from build123d import *

# Parameters (mm, degrees)
SKETCH1_R               = 2
SKETCH1_R_2             = 5.5
SKETCH1_R_3             = 4
BOSS_EXTRUDE1_DEPTH     = 9
BOSS_EXTRUDE2_START     = -27
BOSS_EXTRUDE2_OUTLINE_R = 2
BOSS_EXTRUDE2_DEPTH     = 18
FILLET1_R               = 4
FILLET2_R               = 3
SKETCH3_R               = 11.25
CUT_EXTRUDE1_DEPTH      = 3.5
BOSS_EXTRUDE3_START     = -9
BOSS_EXTRUDE3_DEPTH     = 9
CUT_EXTRUDE2_DEPTH      = 93.793746104
CUT_EXTRUDE2_DEPTH_BACK = 93.793746104
SKETCH7_W               = 7.5
SKETCH7_H               = 5
CUT_EXTRUDE3_DEPTH      = 8.25
SKETCH8_R               = 2
CUT_EXTRUDE5_DEPTH      = 8.25
FILLET4_R               = 6


# Read off the part's stored shape, not the designer's step: Boss-Extrude2
with BuildPart() as part:
    # Sketch1 → Boss-Extrude1 (new body)
    with BuildSketch(Plane.XY):
        with BuildLine():
            Line((0, -15), (55.445040355, -15))
            ThreePointArc((55.445040355, -15), (77.945040355, 7.5), (55.445040355, 30))
            Line((55.445040355, 30), (12.958080577, 30))
            ThreePointArc((12.958080577, 30), (2.222427952, 26.874411477), (-5.157701411, 18.474576271))
            Line((-5.157701411, 18.474576271), (-11.322363742, 5.296610169))
            ThreePointArc((-11.322363742, 5.296610169), (-10.546507173, -6.709782891), (0, -12.5))
            Line((0, -12.5), (0, -15))
        make_face()
        with Locations((50.121730514, 23.802909935)):
            Circle(SKETCH1_R, mode=Mode.SUBTRACT)
        with Locations((60.768350196, -8.802909935)):
            Circle(SKETCH1_R, mode=Mode.SUBTRACT)
        with Locations((55.445040355, 7.5)):
            Circle(SKETCH1_R_2, mode=Mode.SUBTRACT)
        with Locations((71.74795029, 12.823309841)):
            Circle(SKETCH1_R, mode=Mode.SUBTRACT)
        Circle(SKETCH1_R_3, mode=Mode.SUBTRACT)
    extrude(amount=BOSS_EXTRUDE1_DEPTH)

    # Boss-Extrude2 outline → Boss-Extrude2 (add)
    with BuildSketch(Plane.XY.offset(9).offset(BOSS_EXTRUDE2_START)):
        with BuildLine():
            ThreePointArc((55.445040355, -15), (76.903671747, 14.265880489), (42.539570537, 25.930920997))
            Line((42.539570537, 25.930920997), (47.701758465, 18.558552598))
            ThreePointArc((47.701758465, 18.558552598), (68.32021919, 11.559528293), (55.445040355, -6))
            Line((55.445040355, -6), (55.445040355, -15))
        make_face()
        with Locations((60.768350196, -8.802909935)):
            Circle(BOSS_EXTRUDE2_OUTLINE_R, mode=Mode.SUBTRACT)
        with Locations((50.121730514, 23.802909935)):
            Circle(BOSS_EXTRUDE2_OUTLINE_R, mode=Mode.SUBTRACT)
        with Locations((71.74795029, 12.823309841)):
            Circle(BOSS_EXTRUDE2_OUTLINE_R, mode=Mode.SUBTRACT)
    extrude(amount=BOSS_EXTRUDE2_DEPTH)

    # Fillet1
    fillet1_edges = [part.edges().sort_by_distance(p)[0] for p in [
        (55.445040355, -6, -9),
        (55.445040355, -15, -9),
    ]]
    fillet(fillet1_edges, radius=FILLET1_R)

    # Fillet2
    fillet2_edges = [part.edges().sort_by_distance(p)[0] for p in [
        (47.701758465, 18.558552598, -9),
        (42.539570537, 25.930920997, -9),
    ]]
    fillet(fillet2_edges, radius=FILLET2_R)

    # Sketch3 → Cut-Extrude1 (cut)
    with BuildSketch(Plane(origin=(0, 0, 0), x_dir=(-1, 0, 0), z_dir=(0, 0, -1))):
        with Locations((-55.445040355, 7.5)):
            Circle(SKETCH3_R)
    extrude(amount=-CUT_EXTRUDE1_DEPTH, mode=Mode.SUBTRACT)

    # Sketch5 → Boss-Extrude3 (add)
    with BuildSketch(Plane.XY.offset(9).offset(BOSS_EXTRUDE3_START)):
        with BuildLine():
            Line((41.483809243, 30), (41.483809243, 42.5))
            Line((41.483809243, 42.5), (12.958080577, 42.5))
            Line((12.958080577, 42.5), (6.081409657, 42.5))
            Line((6.081409657, 42.5), (-5.157701411, 18.474576271))
            ThreePointArc((-5.157701411, 18.474576271), (2.222427952, 26.874411477), (12.958080577, 30))
            Line((12.958080577, 30), (41.483809243, 30))
        make_face()
    extrude(amount=BOSS_EXTRUDE3_DEPTH)

    # Sketch6 → Cut-Extrude2 (cut, two sides: drawn at the far end of the back side and taken through both)
    with BuildSketch(Plane.XY.offset(9).offset(-CUT_EXTRUDE2_DEPTH_BACK)):
        with BuildLine():
            Line((31.945040355, 28), (31.945040355, 22))
            ThreePointArc((31.945040355, 22), (30.445040355, 20.5), (28.945040355, 22))
            Line((28.945040355, 22), (28.945040355, 28))
            ThreePointArc((28.945040355, 28), (30.445040355, 29.5), (31.945040355, 28))
        make_face()
    extrude(amount=CUT_EXTRUDE2_DEPTH + CUT_EXTRUDE2_DEPTH_BACK, mode=Mode.SUBTRACT)

    # Sketch7 → Cut-Extrude3 (cut)
    with BuildSketch(Plane(origin=(0, 0, 0), x_dir=(-1, 0, 0), z_dir=(0, 0, -1))):
        with Locations((-27.75, -7.5)):
            Rectangle(SKETCH7_W, SKETCH7_H)
        with Locations((-12.75, -7.5)):
            Rectangle(SKETCH7_W, SKETCH7_H)
        with Locations((-42.75, -7.5)):
            Rectangle(SKETCH7_W, SKETCH7_H)
    extrude(amount=-CUT_EXTRUDE3_DEPTH, mode=Mode.SUBTRACT)

    # Sketch8 → Cut-Extrude5 (cut)
    with BuildSketch(Plane.XZ.offset(15)):
        with Locations((42.75, 4.5)):
            Circle(SKETCH8_R)
        with Locations((27.75, 4.5)):
            Circle(SKETCH8_R)
        with Locations((12.75, 4.5)):
            Circle(SKETCH8_R)
    extrude(amount=-CUT_EXTRUDE5_DEPTH, mode=Mode.SUBTRACT)

    # Fillet4
    fillet4_edges = [part.edges().sort_by_distance(p)[0] for p in [
        (41.483809243, 30, 4.5),
        (41.483809243, 42.5, 4.5),
        (6.081409657, 42.5, 4.5),
    ]]
    fillet(fillet4_edges, radius=FILLET4_R)


solid = part.part
The model under review builds one solid part; all positions refer to its coordinate system, in mm. A direction names the side the tool comes from. Round coordinates to 2 decimals unless told otherwise and drop trailing zeros. Loops run counter-clockwise (first coordinate to the right, second up) from the corner with the lowest first, then second, coordinate; pieces in that order, holes last. Notation, with made-up numbers: (-29, 23.25) -> (-2, 23.25) arc R32 cw to (-2, 50.25) -> close; hole circle Ø3 at (-37, 22.5). An arc over 180 degrees is marked (long way). One line per question, with ' | ' between items. Start each with the question number.
Item 1: Add section B-B, the plane y = 8.5. Write out the cut boundary in (x, z), then the cut area to 3 significant figures.
Item 2: Wall thickness on line 1 along Y through (x, z) = (51, 2.5); line 2 along Z through (x, y) = (12.75, -12.75); line 3 along Z through (x, y) = (6.5, 19): over which ranges is each line inside the solid? List them lowest first. Write a range as [from, to].
Item 3: Add section A-A, the plane x = 27.75. Write out the cut boundary in (y, z), then the cut area to 3 significant figures.
Item 4: Add section D-D, the plane x = 42.75. Write out the cut boundary in (y, z).
Item 5: Draft analysis for pull direction Y (two halves, no side actions). For faces 6 (the face through (39, -8, 4)), 7 (the face through (39.77, 40.7, 4.56)), 8 (the face through (56.98, -13.713, -8.874)), state which applies: +Y half, -Y half, draft (parallel to the pull), parting line (faces both ways), or undercut.
Item 6: For pin 1 (9 mm diameter, centred on x = 0, y = 0, fed in from +Z); pin 2 (18 mm diameter, centred on x = 55.45, y = 7.5, fed in from -Z); pin 3 (12 mm diameter, centred on y = -6.5, z = -2, fed in from -X); pin 4 (11 mm diameter, centred on x = 52, y = 2.5, fed in from -Z), all flat-tipped, find the tip position at first contact; note any pin that passes through.
Item 7: Machinability: for faces 1 (the face through (30.5, 20.5, 4.4)), 2 (the face through (31.5, -8, 4)), 3 (the face through (11.163, -12.535, 3.283)), 4 (the face through (52, 30, 4)), 5 (the face through (47.78, 19.625, -8.874)), which of the approach directions +Z, -Z, +X, -X, +Y, -Y give a long, thin tool a straight path to every point of the face, cutting with its end or side? Answer none if there is none.
Item 8: Add section C-C, the plane z = -11.75. Write out the cut boundary in (x, y), then the cut area to 3 significant figures.
Return value:
1) outline: (-9.82, 0) -> (44.24, 0) -> (44.24, 3.5) -> (50.04, 3.5) -> (50.04, 9) -> (-9.82, 9) -> close; (60.85, 3.5) -> (66.65, 3.5) -> (66.65, 0) -> (68.91, 0) -> (68.91, -18) -> (77.92, -18) -> (77.92, 9) -> (60.85, 9) -> close | area: 814 mm2
2) line 1: y = [-15, -2.83], [17.83, 22.01], [25.6, 30] | line 2: z = [0, 2.5], [6.5, 9] | line 3: z = [0, 9]
3) outline: (-15, 0) -> (-10, 0) -> (-10, 2.5) -> (-15, 2.5) -> close; (-15, 6.5) -> (-10, 6.5) -> (-10, 8.25) -> (-5, 8.25) -> (-5, 0) -> (42.5, 0) -> (42.5, 9) -> (-15, 9) -> close | area: 456 mm2
4) outline: (-15, 0) -> (-10, 0) -> (-10, 2.5) -> (-15, 2.5) -> close; (-15, 6.5) -> (-10, 6.5) -> (-10, 8.25) -> (-5, 8.25) -> (-5, 0) -> (32.31, 0) -> (32.31, 9) -> (-15, 9) -> close
5) face 6: undercut | face 7: +Y half | face 8: -Y half
6) pin 1: stops at z = 9 | pin 2: stops at z = 3.5 | pin 3: stops at x = -12.47 | pin 4: stops at z = 0
7) face 1: +Z, -Z | face 2: -Z | face 3: -Y | face 4: +Z, -Z, +X, +Y | face 5: -Z, -Y
8) outline: (44.39, 23.28) -> (46.14, 20.79) arc R3 ccw to (49.84, 19.78) arc R13.5 cw (long way) to (58.53, -5.64) arc R4 ccw to (55.45, -9.54) -> (55.45, -10.56) arc R4 ccw to (60.31, -14.47) arc R22.5 ccw (long way) to (45.53, 27.7) arc R3 ccw to start; hole circle Ø4 at (50.12, 23.8); hole circle Ø4 at (60.77, -8.8); hole circle Ø4 at (71.75, 12.82) | area: 559 mm2
